Design review of the part built by this model. Coordinates are the model's own, in mm. Coordinates: 2 decimals unless noted, no trailing zeros. Write each loop counter-clockwise with the first axis right and the second up, starting at its lowest first coordinate (ties: lowest second). Pieces come first, ordered by that corner, then holes. Notation, with made-up numbers: (89, 80.25) -> (95, 80.25) arc R13 ccw to (95, 98.25) -> close; hole circle Ø5 at (79, 30). An arc over 180 degrees is marked (long way). One line per question, with ' | ' between items. Start each with the question number.
Q1. Add section D-D on y = 2.05. State the section outline as (x, z) points.
Q2. For P1, Ø1.5, axis at x = 30.5, y = 2, coming from the -Z side; P2, Ø1.5, axis at x = 29.5, y = 2, coming from the -Z side; P3, Ø1.5, axis at x = -34.5, y = 1, coming from the -Z side, all flat-tipped, find the tip position at first contact; note any pin that passes through.
Q3. Add section C-C on z = 18.5. State the section outline as (x, y) points.
Q4. Add section B-B on x = -9. State the section outline as (y, z) points (3 decimals).
Q5. Wall thickness on probe 1 along X at (y, z) = (0.45, 22); probe 2 along X at (y, z) = (1, -12.5); probe 3 along Z at (x, y) = (-45, 1.55): over which ranges is each line inside the solid? List them lowest first.
Q6. Add section A-A on z = -5. State the section outline as (x, y) points, and give its area (3 significant figures).
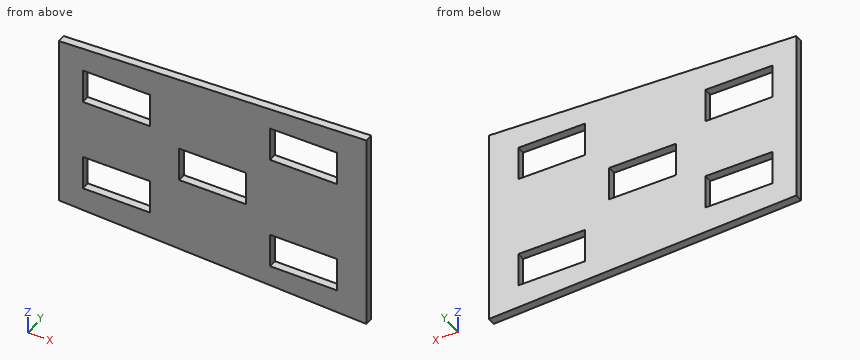
from build123d import *

# Parameters (mm, degrees)
BOSS_EXTRUDE1_DEPTH = 3
SKETCH2_W           = 25
SKETCH2_H           = 13
CUT_EXTRUDE1_DEPTH  = 3


with BuildPart() as part:
    # Sketch1 → Boss-Extrude1 (new body)
    with BuildSketch(Plane(origin=(0, 0, 0), x_dir=(1, 0, 0), z_dir=(0, 1, 0))):
        Polygon((-57.5, -33.023654191), (57.5, -37.976345809), (57.5, 38.023654191), (-57.5, 32.976345809), align=None)
    extrude(amount=BOSS_EXTRUDE1_DEPTH)

    # Sketch2 → Cut-Extrude1 (cut)
    with BuildSketch(Plane(origin=(0, 3, 0), x_dir=(1, 0, 0), z_dir=(0, 1, 0))):
        with Locations((34, -21.994267552)):
            Rectangle(SKETCH2_W, SKETCH2_H)
        Rectangle(SKETCH2_W, SKETCH2_H)
        with Locations((-36, -17.902913606)):
            Rectangle(SKETCH2_W, SKETCH2_H)
        with Locations((-36, 17.862688371)):
            Rectangle(SKETCH2_W, SKETCH2_H)
        with Locations((34, 22.032203991)):
            Rectangle(SKETCH2_W, SKETCH2_H)
    extrude(amount=-CUT_EXTRUDE1_DEPTH, mode=Mode.SUBTRACT)


solid = part.part
Output values:
1) outline: (-57.5, -32.98) -> (57.5, -38.02) -> (57.5, 37.98) -> (-57.5, 33.02) -> close; hole (-48.5, -24.36) -> (-23.5, -24.36) -> (-23.5, -11.36) -> (-48.5, -11.36) -> close; hole (-48.5, 11.4) -> (-23.5, 11.4) -> (-23.5, 24.4) -> (-48.5, 24.4) -> close; hole (-12.5, -6.5) -> (12.5, -6.5) -> (12.5, 6.5) -> (-12.5, 6.5) -> close; hole (21.5, -28.53) -> (46.5, -28.53) -> (46.5, -15.53) -> (21.5, -15.53) -> close; hole (21.5, 15.49) -> (46.5, 15.49) -> (46.5, 28.49) -> (21.5, 28.49) -> close
2) P1: stops at z = -36.87 | P2: stops at z = -36.83 | P3: stops at z = -34.02
3) outline: (-57.5, 0) -> (-48.5, 0) -> (-48.5, 3) -> (-57.5, 3) -> close; (-23.5, 0) -> (21.5, 0) -> (21.5, 3) -> (-23.5, 3) -> close; (46.5, 0) -> (57.5, 0) -> (57.5, 3) -> (46.5, 3) -> close
4) outline: (0, -35.105) -> (3, -35.105) -> (3, -6.5) -> (0, -6.5) -> close; (0, 6.5) -> (3, 6.5) -> (3, 35.112) -> (0, 35.112) -> close
5) probe 1: x = -57.5 to -48.5, -23.5 to 21.5, 46.5 to 57.5 | probe 2: x = -57.5 to -48.5, -23.5 to 57.5 | probe 3: z = -33.52 to -24.36, -11.36 to 11.4, 24.4 to 33.56
6) outline: (-57.5, 0) -> (-12.5, 0) -> (-12.5, 3) -> (-57.5, 3) -> close; (12.5, 0) -> (57.5, 0) -> (57.5, 3) -> (12.5, 3) -> close | area: 270 mm2
